Model file for the job. Use its own axes, mm. A direction names the side the tool comes from. Give positions to 0.01 mm unless a question says otherwise; leave off trailing zeros. Loops run counter-clockwise (first coordinate to the right, second up) from the corner with the lowest first, then second, coordinate; pieces in that order, holes last. Notation, with made-up numbers: (-17, -31.5) - (18, -31.5) arc R19 cw to (18, -21.5) - close; hole circle Ø2 at (29.25, 87). An arc over 180 degrees is marked (long way). Answer as CSV lines item,"result". Start each with the question number.
Item 1: Pin check, flat tip, straight feed: pin 1 (2.5 mm diameter, centred on y = 875, z = 0, fed in from +X). Stop position of the tip, or through.
Item 2: Saw through at A-A on y = 505.5. Give the cut face in (x, z), plus the area to 3 significant figures.
Item 3: Pull direction Z, two halves, no side cores. Call faces 1 (the flat face through (14, 492, 0)), 2 (the flat face through (0, 492, -10)), 3 (the cylindrical face through (-1.63, 46.93, 9.51)): pulls with the +Z half, pulls with the -Z half, needs draft (parallel to the pull), parting line crosses it, or undercut.
Item 4: Drill centre lines: L1, parallel to Z at x = -13.25, y = 658; L2, parallel to X at y = 521, z = 8.5; L3, parallel to Z at x = -14.4, y = 595. Where is each one in solid material? Low to high. Write a range as from..to.
Item 5: Tool access for faces 4 (the flat face through (-14, 492, 0)), 5 (the flat face through (15, 492, 0)): list every direction of +Z, -Z, +X, -X, +Y, -Y with a clear straight run to the whole face (end or side of a thin tool).
from build123d import *

# Parameters (mm, degrees)
SKETCH_1_W           = 30
SKETCH_1_H           = 20
SKETCH_1_W_2         = 28
SKETCH_1_H_2         = 18
EXTRUDE_1_DEPTH      = 980
CUT_EXTRUDE_3_DEPTH  = 981.51007134
SKETCH_5_W           = 15
SKETCH_5_H           = 12
CUT_EXTRUDE_4_DEPTH  = 10
SKETCH_9_R           = 1.5
CUT_EXTRUDE_7_DEPTH  = 981.318825689
SKETCH_13_W          = 30
SKETCH_13_H          = 20
SKETCH_13_W_2        = 28
SKETCH_13_H_2        = 18
EXTRUDE_2_DEPTH      = 10
CUT_EXTRUDE_8_DEPTH  = 60
SKETCH_15_W          = 15
SKETCH_15_H          = 15
CUT_EXTRUDE_10_DEPTH = 5
FILLET_1_R           = 2
SKETCH_16_R          = 2
CUT_EXTRUDE_11_DEPTH = 90
FILLET_2_R           = 2
SKETCH_17_R          = 1.5
CUT_EXTRUDE_12_DEPTH = 40
CUT_EXTRUDE_15_DEPTH = 51
SKETCH_21_W          = 22.187259215
SKETCH_21_H          = 65.33837704
EXTRUDE_3_DEPTH      = 1
SKETCH_22_R          = 1.65
CUT_EXTRUDE_16_DEPTH = 1
SKETCH_23_R          = 7.5
CUT_EXTRUDE_17_DEPTH = 10


with BuildPart() as part:
    # Sketch 1 → Extrude 1 (new body)
    with BuildSketch(Plane(origin=(0, 0, 0), x_dir=(1, 0, 0), z_dir=(0, 1, 0))):
        Rectangle(SKETCH_1_W, SKETCH_1_H)
        Rectangle(SKETCH_1_W_2, SKETCH_1_H_2, mode=Mode.SUBTRACT)
    extrude(amount=EXTRUDE_1_DEPTH)

    # Sketch 4 → Cut-Extrude 3 (cut, through all)
    with BuildSketch(Plane(origin=(15, 0, 0), x_dir=(0, 0, -1), z_dir=(1, 0, 0))):
        with BuildLine():
            Line((3.4, 968), (3.4, 972))
            ThreePointArc((3.4, 972), (5, 973.6), (6.6, 972))
            Line((6.6, 972), (6.6, 968))
            ThreePointArc((6.6, 968), (5, 966.4), (3.4, 968))
        make_face()
        with BuildLine():
            Line((-3.4, 968), (-3.4, 972))
            ThreePointArc((-3.4, 972), (-5, 973.6), (-6.6, 972))
            Line((-6.6, 972), (-6.6, 968))
            ThreePointArc((-6.6, 968), (-5, 966.4), (-3.4, 968))
        make_face()
    extrude(amount=-CUT_EXTRUDE_3_DEPTH, mode=Mode.SUBTRACT)

    # Sketch 5 → Cut-Extrude 4 (cut)
    with BuildSketch(Plane(origin=(15, 0, 0), x_dir=(0, 0, -1), z_dir=(1, 0, 0))):
        with Locations((0, 968)):
            Rectangle(SKETCH_5_W, SKETCH_5_H)
    extrude(amount=-CUT_EXTRUDE_4_DEPTH, mode=Mode.SUBTRACT)

    # Sketch 9 → Cut-Extrude 7 (cut, through all)
    with BuildSketch(Plane.XY.offset(10)):
        with Locations((11, 977)):
            Circle(SKETCH_9_R)
        with Locations(Location((-11, 977, 0), (0, 0, 180))):
            Circle(SKETCH_9_R)
    extrude(amount=-CUT_EXTRUDE_7_DEPTH, mode=Mode.SUBTRACT)

    # Sketch 13 → Extrude 2 (add)
    with BuildSketch(Plane.XZ):
        Rectangle(SKETCH_13_W, SKETCH_13_H)
        Rectangle(SKETCH_13_W_2, SKETCH_13_H_2, mode=Mode.SUBTRACT)
    extrude(amount=EXTRUDE_2_DEPTH)

    # Sketch 11 → Cut-Extrude 8 (cut)
    with BuildSketch(Plane(origin=(-14, 0, 0), x_dir=(0, 0, -1), z_dir=(1, 0, 0))):
        with BuildLine():
            Line((-6.6, 5), (-6.6, 15))
            ThreePointArc((-6.6, 15), (-5, 16.6), (-3.4, 15))
            Line((-3.4, 15), (-3.4, 5))
            ThreePointArc((-3.4, 5), (-5, 3.4), (-6.6, 5))
        make_face()
        with BuildLine():
            Line((6.6, 5), (6.6, 15))
            ThreePointArc((6.6, 15), (5, 16.6), (3.4, 15))
            Line((3.4, 15), (3.4, 5))
            ThreePointArc((3.4, 5), (5, 3.4), (6.6, 5))
        make_face()
    extrude(amount=-CUT_EXTRUDE_8_DEPTH, mode=Mode.SUBTRACT)

    # Sketch 15 → Cut-Extrude 10 (cut)
    with BuildSketch(Plane(origin=(15, 0, 0), x_dir=(0, 0, -1), z_dir=(1, 0, 0))):
        with Locations((0, 10)):
            Rectangle(SKETCH_15_W, SKETCH_15_H)
    extrude(amount=-CUT_EXTRUDE_10_DEPTH, mode=Mode.SUBTRACT)

    # Fillet 1
    fillet_1_edges = [part.edges().sort_by_distance(p)[0] for p in [
        (14.5, 17.5, -7.5),
        (14.5, 2.5, -7.5),
        (14.5, 2.5, 7.5),
        (14.5, 17.5, 7.5),
    ]]
    fillet(fillet_1_edges, radius=FILLET_1_R)

    # Sketch 16 → Cut-Extrude 11 (cut)
    with BuildSketch(Plane.XY.offset(10)):
        with Locations((10, 21)):
            Circle(SKETCH_16_R)
        with Locations((0, 21)):
            Circle(SKETCH_16_R)
        with Locations((-10, 21)):
            Circle(SKETCH_16_R)
    extrude(amount=-CUT_EXTRUDE_11_DEPTH, mode=Mode.SUBTRACT)

    # Fillet 2
    fillet_2_edges = [part.edges().sort_by_distance(p)[0] for p in [
        (14.5, 974, -7.5),
        (14.5, 962, -7.5),
        (14.5, 962, 7.5),
        (14.5, 974, 7.5),
    ]]
    fillet(fillet_2_edges, radius=FILLET_2_R)

    # Sketch 17 → Cut-Extrude 12 (cut)
    with BuildSketch(Plane(origin=(15, 0, 0), x_dir=(0, 0, -1), z_dir=(1, 0, 0))):
        with Locations((0, 955)):
            Circle(SKETCH_17_R)
        with Locations((0, 915)):
            Circle(SKETCH_17_R)
        with Locations((0, 875)):
            Circle(SKETCH_17_R)
        with Locations((0, 835)):
            Circle(SKETCH_17_R)
        with Locations((0, 795)):
            Circle(SKETCH_17_R)
        with Locations((0, 755)):
            Circle(SKETCH_17_R)
        with Locations((0, 715)):
            Circle(SKETCH_17_R)
        with Locations((0, 675)):
            Circle(SKETCH_17_R)
        with Locations((0, 635)):
            Circle(SKETCH_17_R)
        with Locations((0, 595)):
            Circle(SKETCH_17_R)
        with Locations((0, 555)):
            Circle(SKETCH_17_R)
        with Locations((0, 515)):
            Circle(SKETCH_17_R)
        with Locations((0, 475)):
            Circle(SKETCH_17_R)
        with Locations((0, 435)):
            Circle(SKETCH_17_R)
        with Locations((0, 395)):
            Circle(SKETCH_17_R)
        with Locations((0, 355)):
            Circle(SKETCH_17_R)
        with Locations((0, 315)):
            Circle(SKETCH_17_R)
        with Locations((0, 275)):
            Circle(SKETCH_17_R)
        with Locations((0, 235)):
            Circle(SKETCH_17_R)
        with Locations((0, 195)):
            Circle(SKETCH_17_R)
        with Locations((0, 155)):
            Circle(SKETCH_17_R)
        with Locations((0, 115)):
            Circle(SKETCH_17_R)
        with Locations((0, 75)):
            Circle(SKETCH_17_R)
        with Locations((0, 35)):
            Circle(SKETCH_17_R)
    extrude(amount=-CUT_EXTRUDE_12_DEPTH, mode=Mode.SUBTRACT)

    # Sketch 20 → Cut-Extrude 15 (cut)
    with BuildSketch(Plane(origin=(15, 0, 0), x_dir=(0, 0, -1), z_dir=(1, 0, 0))):
        with BuildLine():
            Line((-6, 50), (-6, 100))
            ThreePointArc((-6, 100), (0, 106), (6, 100))
            Line((6, 100), (6, 50))
            ThreePointArc((6, 50), (0, 44), (-6, 50))
        make_face()
    extrude(amount=-CUT_EXTRUDE_15_DEPTH, mode=Mode.SUBTRACT)

    # Sketch 21 → Extrude 3 (add)
    with BuildSketch(Plane.XY.offset(10)):
        with Locations((-0.689634309, 76.201822832)):
            Rectangle(SKETCH_21_W, SKETCH_21_H)
    extrude(amount=-EXTRUDE_3_DEPTH)

    # Sketch 22 → Cut-Extrude 16 (cut)
    with BuildSketch(Plane.XY.offset(10)):
        with Locations((5, 40)):
            Circle(SKETCH_22_R)
        with Locations((-5, 40)):
            Circle(SKETCH_22_R)
        with Locations((5, 88)):
            Circle(SKETCH_22_R)
        with Locations((-5, 88)):
            Circle(SKETCH_22_R)
    extrude(amount=-CUT_EXTRUDE_16_DEPTH, mode=Mode.SUBTRACT)

    # Sketch 23 → Cut-Extrude 17 (cut)
    with BuildSketch(Plane.XY.offset(10)):
        with Locations((0, 54.25)):
            Circle(SKETCH_23_R)
    extrude(amount=-CUT_EXTRUDE_17_DEPTH, mode=Mode.SUBTRACT)


solid = part.part
Responses:
1,pin 1,"through"
2,outline,"(-15, -10) - (15, -10) - (15, 10) - (-15, 10) - close; hole (-14, -9) - (14, -9) - (14, 9) - (-14, 9) - close"
2,area,"96.0 mm2"
3,face 1,"undercut"
3,face 2,"pulls with the -Z half"
3,face 3,"needs draft"
4,L1,"-10..-9, 9..10"
4,L2,"-15..-14, 14..15"
4,L3,"-10..-1.5, 1.5..10"
5,face 4,"+Y, -Y"
5,face 5,"+Z, -Z, +X, +Y, -Y"
